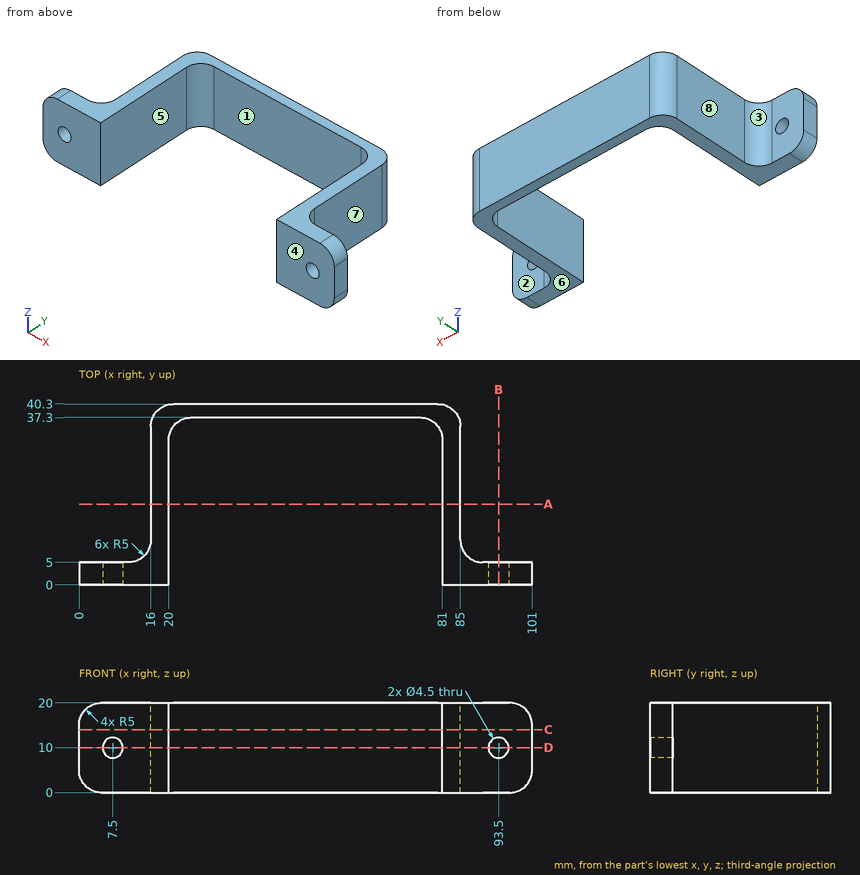
For this review, use the dimensioned drawing (mm, ordinates from the lowest corner) and the shaded views. A direction names the side the tool comes from. Give positions to 0.01 mm unless a question says otherwise; leave off trailing zeros. Loops run counter-clockwise (first coordinate to the right, second up) from the corner with the lowest first, then second, coordinate; pieces in that order, holes last.
Item 1: Take a section at C-C, the plane z = 14. State the section outline as (x, y) points.
Item 2: Insertion check: pin 1 (10 mm diameter, centred on y = 13, z = 12, fed in from -X); pin 2 (9 mm diameter, centred on x = 3.5, z = 7.5, fed in from +Y); pin 3 (9 mm diameter, centred on x = 93, z = 14, fed in from +Y); pin 4 (7 mm diameter, centred on x = 93.5, z = 10, fed in from -Y). Each pin has a flat end and moves straight along its axis. Give the tip position at first contact, or say it passes through.
Item 3: Take a section at D-D, the plane z = 10. State the section outline as (x, y) points, and give its area (3 significant figures).
Item 4: Tool access review of the marked faces 4, 5, 6, 7 and 8: name each direction out of +Z, -Z, +X, -X, +Y, -Y from which nothing blocks a thin tool from reaching the whole face with its end or side.
Item 5: Take a section at A-A, the plane y = 18. State the section outline as (x, z) points.
Item 6: For line 1 along Z through (x, y) = (7.5, 3.4); line 2 along X through (y, z) = (13.5, 10.75); line 3 along Y through (x, z) = (72.5, 4), list the stretches that pass through material, from the lowest coordinate up.
Item 7: Draft analysis for pull direction X (two halves, no side actions). For the marked faces 1, 2 and 3, state which applies: +X half, -X half, draft (parallel to the pull), parting line (faces both ways), or undercut.
Item 8: Take a section at B-B, the plane x = 93.5. State the section outline as (y, z) points, and give its area (3 significant figures).
Calculated:
1. outline: (0, 0) - (20, 0) - (20, 32.3) arc R5 cw to (25, 37.3) - (76, 37.3) arc R5 cw to (81, 32.3) - (81, 0) - (101, 0) - (101, 5) - (90, 5) arc R5 cw to (85, 10) - (85, 35.3) arc R5 ccw to (80, 40.3) - (21, 40.3) arc R5 ccw to (16, 35.3) - (16, 10) arc R5 cw to (11, 5) - (0, 5) - close
2. pin 1: stops at x = 15.58
2. pin 2: stops at y = 5
2. pin 3: stops at y = 5.23
2. pin 4: stops at y = 0
3. outline: (0, 0) - (5.25, 0) - (5.25, 5) - (0, 5) - close; (9.75, 0) - (20, 0) - (20, 32.3) arc R5 cw to (25, 37.3) - (76, 37.3) arc R5 cw to (81, 32.3) - (81, 0) - (91.25, 0) - (91.25, 5) - (90, 5) arc R5 cw to (85, 10) - (85, 35.3) arc R5 ccw to (80, 40.3) - (21, 40.3) arc R5 ccw to (16, 35.3) - (16, 10) arc R5 cw to (11, 5) - (9.75, 5) - close; (95.75, 0) - (101, 0) - (101, 5) - (95.75, 5) - close
3. area: 631 mm2
4. face 4: +Z, -Z, +X, -X, -Y
4. face 5: +Z, -Z, -Y
4. face 6: -Z, +X, -X, +Y, -Y
4. face 7: +Z, -Z, +X, +Y
4. face 8: +Z, -Z, -X, +Y
5. outline: (16, 0) - (20, 0) - (20, 20) - (16, 20) - close; (81, 0) - (85, 0) - (85, 20) - (81, 20) - close
6. line 1: z = 0 to 7.75, 12.25 to 20
6. line 2: x = 16 to 20, 81 to 85
6. line 3: y = 37.3 to 40.3
7. face 1: undercut
7. face 2: draft
7. face 3: -X half
8. outline: (0, 0) - (5, 0) - (5, 7.75) - (0, 7.75) - close; (0, 12.25) - (5, 12.25) - (5, 20) - (0, 20) - close
8. area: 77.5 mm2
